Verification items for the finished model (mm, model axes). Give positions to 0.01 mm unless a question says otherwise; leave off trailing zeros. Write each loop counter-clockwise with the first axis right and the second up, starting at its lowest first coordinate (ties: lowest second). Pieces come first, ordered by that corner, then holes. Notation, with made-up numbers: (84.25, 58) -> (108.25, 58) arc R21 ccw to (108.25, 89) -> close; hole circle Ø7 at (-24.5, 41). An arc over 180 degrees is marked (long way). Write item = value, one per line.
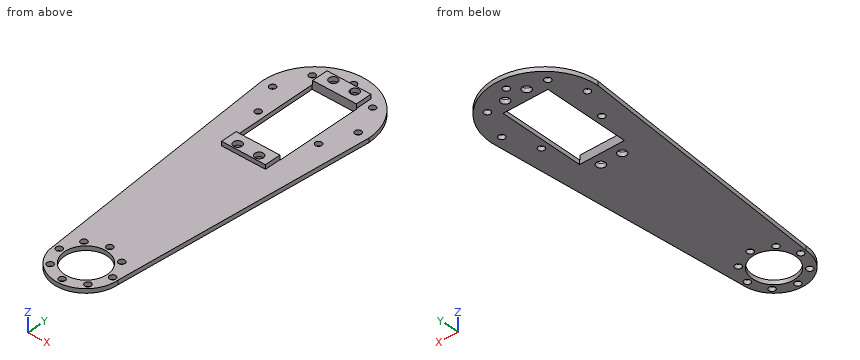
from build123d import *

# Parameters (mm, degrees)
SKETCH_1_W          = 20.5
SKETCH_1_H          = 15.141704846
SKETCH_1_R          = 2
EXTRUDE_1_DEPTH     = 29
SKETCH_2_W          = 20.5
SKETCH_2_H          = 70.283409692
EXTRUDE_2_DEPTH     = 3
SKETCH_3_W          = 20.5
SKETCH_3_H          = 7.570852423
CUT_EXTRUDE_1_DEPTH = 49.621002864
SKETCH_5_R          = 2.5
EXTRUDE_3_DEPTH     = 10
CUT_EXTRUDE_2_REACH = 75.297
SKETCH_8_R          = 1.6
SKETCH_9_W          = 20.5
SKETCH_9_H          = 55.141704846
CUT_EXTRUDE_3_DEPTH = 30
SKETCH_11_R         = 2.5
CUT_EXTRUDE_4_DEPTH = 10
SKETCH_12_W         = 21
SKETCH_12_H         = 40
SKETCH_12_R         = 2
EXTRUDE_5_DEPTH     = 2
SKETCH_13_R         = 10
CUT_EXTRUDE_5_DEPTH = 2
SKETCH_14_R         = 1.5
CUT_EXTRUDE_6_DEPTH = 128.538229563


with BuildPart() as part:
    # Sketch 1 → Extrude 1 (new body)
    # profile 1 of 3: a face of its own
    with BuildSketch(Plane.XY):
        with BuildLine():
            Line((-10.25, 35.141704846), (-10.25, 20))
            Line((-10.25, 20), (-5, 20))
            Line((-5, 20), (-5, 23))
            ThreePointArc((-5, 23), (-6.414213562, 26.414213562), (-3, 25))
            Line((-3, 25), (3, 25))
            ThreePointArc((3, 25), (5, 27), (7, 25))
            ThreePointArc((7, 25), (6.414213562, 23.585786438), (5, 23))
            Line((5, 23), (5, 20))
            Line((5, 20), (10.25, 20))
            Line((10.25, 20), (10.25, 35.141704846))
            Line((10.25, 35.141704846), (-10.25, 35.141704846))
        make_face()
    # profile 2 of 3: a face of its own
    with BuildSketch(Plane.XY):
        with Locations((0, -27.570852423)):
            Rectangle(SKETCH_1_W, SKETCH_1_H)
        with Locations(Location((-5, -25, 0), (0, 0, 180))):
            Circle(SKETCH_1_R, mode=Mode.SUBTRACT)
        with Locations(Location((5, -25, 0), (0, 0, 180))):
            Circle(SKETCH_1_R, mode=Mode.SUBTRACT)
    # profile 3 of 3: a face of its own
    with BuildSketch(Plane.XY):
        with BuildLine():
            Line((-5, 23), (-5, 20))
            Line((-5, 20), (5, 20))
            Line((5, 20), (5, 23))
            ThreePointArc((5, 23), (3.585786438, 23.585786438), (3, 25))
            Line((3, 25), (-3, 25))
            ThreePointArc((-3, 25), (-3.585786438, 23.585786438), (-5, 23))
        make_face()
    extrude(amount=EXTRUDE_1_DEPTH)

    # Sketch 2 → Extrude 2 (add)
    with BuildSketch(Plane.XY.offset(29)):
        Rectangle(SKETCH_2_W, SKETCH_2_H)
    extrude(amount=EXTRUDE_2_DEPTH)

    # Sketch 3 → Cut-Extrude 1 (cut, through all)
    with BuildSketch(Plane(origin=(0, 0, 0), x_dir=(-1, 0, 0), z_dir=(0, 0, -1))):
        with Locations((0, -31.356278635)):
            Rectangle(SKETCH_3_W, SKETCH_3_H)
        with Locations((0, 31.356278635)):
            Rectangle(SKETCH_3_W, SKETCH_3_H)
    extrude(amount=-CUT_EXTRUDE_1_DEPTH, mode=Mode.SUBTRACT)

    # Sketch 5 → Extrude 3 (add)
    with BuildSketch(Plane.XZ.offset(27.570852423)):
        with Locations(Location((0, 2.5, 0), (0, 0, 270))):
            Circle(SKETCH_5_R)
    extrude(amount=EXTRUDE_3_DEPTH)

    # Sketch 8 → Cut-Extrude 2 (cut, up to next)
    with BuildSketch(Plane(origin=(0, 27.570852423, 0), x_dir=(1, 0, 0), z_dir=(0, 1, 0)), mode=Mode.PRIVATE) as cut_extrude_2_sk1:
        with Locations(Location((0, -16.5, 0), (0, 0, 270))):
            Circle(SKETCH_8_R)
    cut_extrude_2_tool1 = extrude(cut_extrude_2_sk1.sketch, amount=-CUT_EXTRUDE_2_REACH, mode=Mode.PRIVATE) & part.part
    # Sketch 8 → Cut-Extrude 2 (cut, up to next)
    with BuildSketch(Plane(origin=(0, 27.570852423, 0), x_dir=(1, 0, 0), z_dir=(0, 1, 0)), mode=Mode.PRIVATE) as cut_extrude_2_sk2:
        with Locations(Location((0, -26.5, 0), (0, 0, 270))):
            Circle(SKETCH_8_R)
    cut_extrude_2_tool2 = extrude(cut_extrude_2_sk2.sketch, amount=-CUT_EXTRUDE_2_REACH, mode=Mode.PRIVATE) & part.part
    add(cut_extrude_2_tool1.solids().sort_by_distance((0, 27.570852, 16.5))[0], mode=Mode.SUBTRACT)
    add(cut_extrude_2_tool2.solids().sort_by_distance((0, 27.570852, 26.5))[0], mode=Mode.SUBTRACT)

    # Sketch 9 → Cut-Extrude 3 (cut)
    with BuildSketch(Plane.XY.offset(32)):
        Rectangle(SKETCH_9_W, SKETCH_9_H)
    extrude(amount=-CUT_EXTRUDE_3_DEPTH, mode=Mode.SUBTRACT)


with BuildPart() as cut_extrude_3_piece_1:
    # of the separate pieces the step leaves, piece 1, a body of its own (cut_extrude_3_pieces)
    add(part.part.solids().sort_by_distance((10.25, -20, 2))[0])

    # Sketch 11 → Cut-Extrude 4 (cut)
    with BuildSketch(Plane.XZ.offset(37.570852423)):
        with Locations((0, 2.5)):
            Circle(SKETCH_11_R)
    extrude(amount=-CUT_EXTRUDE_4_DEPTH, mode=Mode.SUBTRACT)



with BuildPart() as cut_extrude_3_piece_2:
    # of the separate pieces the step leaves, piece 2, a body of its own (cut_extrude_3_pieces)
    add(part.part.solids().sort_by_distance((10.25, 20, 0))[0])


with BuildPart() as cut_extrude_3_piece_1_1:
    add(cut_extrude_3_piece_1.part)

    add(cut_extrude_3_piece_2.part)  # Extrude 5 merges Cut-Extrude 3 piece 2
    # Sketch 12 → Extrude 5 (add)
    with BuildSketch(Plane(origin=(0, 0, 0), x_dir=(-1, 0, 0), z_dir=(0, 0, -1))):
        with BuildLine():
            Line((15, -110), (25, 10))
            ThreePointArc((25, 10), (0, 35), (-25, 10))
            Line((-25, 10), (-15, -110))
            ThreePointArc((-15, -110), (0, -125), (15, -110))
        make_face()
        Rectangle(SKETCH_12_W, SKETCH_12_H, mode=Mode.SUBTRACT)
        with Locations((-5, 25)):
            Circle(SKETCH_12_R, mode=Mode.SUBTRACT)
        with Locations((5, 25)):
            Circle(SKETCH_12_R, mode=Mode.SUBTRACT)
        with Locations(Location((5, -25, 0), (0, 0, 180))):
            Circle(SKETCH_12_R, mode=Mode.SUBTRACT)
        with Locations(Location((-5, -25, 0), (0, 0, 180))):
            Circle(SKETCH_12_R, mode=Mode.SUBTRACT)
    extrude(amount=EXTRUDE_5_DEPTH)

    # Sketch 13 → Cut-Extrude 5 (cut)
    with BuildSketch(Plane(origin=(0, 0, -2), x_dir=(-1, 0, 0), z_dir=(0, 0, -1))):
        with Locations((0, -110)):
            Circle(SKETCH_13_R)
    extrude(amount=-CUT_EXTRUDE_5_DEPTH, mode=Mode.SUBTRACT)

    # Sketch 14 → Cut-Extrude 6 (cut, through all)
    with BuildSketch(Plane(origin=(0, 0, -2), x_dir=(-1, 0, 0), z_dir=(0, 0, -1))):
        with Locations((-20, 10)):
            Circle(SKETCH_14_R)
        with Locations((-14.142135624, 24.142135624)):
            Circle(SKETCH_14_R)
        with Locations((0, 30)):
            Circle(SKETCH_14_R)
        with Locations((14.142135624, 24.142135624)):
            Circle(SKETCH_14_R)
        with Locations((20, 10)):
            Circle(SKETCH_14_R)
        with Locations((14.142135624, -4.142135624)):
            Circle(SKETCH_14_R)
        with Locations((-14.142135624, -4.142135624)):
            Circle(SKETCH_14_R)
        with Locations((0, -97.5)):
            Circle(SKETCH_14_R)
        with Locations((8.838834765, -101.161165235)):
            Circle(SKETCH_14_R)
        with Locations((12.5, -110)):
            Circle(SKETCH_14_R)
        with Locations((8.838834765, -118.838834765)):
            Circle(SKETCH_14_R)
        with Locations((0, -122.5)):
            Circle(SKETCH_14_R)
        with Locations((-8.838834765, -118.838834765)):
            Circle(SKETCH_14_R)
        with Locations((-12.5, -110)):
            Circle(SKETCH_14_R)
        with Locations((-8.838834765, -101.161165235)):
            Circle(SKETCH_14_R)
    extrude(amount=-CUT_EXTRUDE_6_DEPTH, mode=Mode.SUBTRACT)


solid = cut_extrude_3_piece_1_1.part
Item 1: Material ranges on line 1 (Y direction, x = 5, z = 0.8); line 2 (Y direction, x = 0, z = -1.2); line 3 (X direction, y = -24, z = -1.75), recorded low to high.
Response values:
line_1 = -27.57 to -27, -23 to -20, 20 to 23, 27 to 27.57
line_2 = -125 to -124, -121 to -120, -100 to -99, -96 to -20, 20 to 28.5, 31.5 to 35
line_3 = -22.17 to -6.73, -3.27 to 3.27, 6.73 to 22.17
Item 2: Sectioned sample at D-D on z = -0.75. Give the number of separate pieces and of enclosed holes in the cut face, then the cut area to 3 significant figures.
Response values:
separate_pieces = 1
enclosed_holes = 21
area = 4,820 mm^2
Item 3: Sectioned sample at A-A on x = 0. Record the cut outline in (y, z), then the cut area to 3 significant figures.
Response values:
outline = (-125, -2) -> (-124, -2) -> (-124, 0) -> (-125, 0) -> close; (-121, -2) -> (-120, -2) -> (-120, 0) -> (-121, 0) -> close; (-100, -2) -> (-99, -2) -> (-99, 0) -> (-100, 0) -> close; (-96, -2) -> (-20, -2) -> (-20, 2) -> (-27.57, 2) -> (-27.57, 0) -> (-96, 0) -> close; (20, -2) -> (28.5, -2) -> (28.5, 0) -> (27.57, 0) -> (27.57, 2) -> (20, 2) -> close; (31.5, -2) -> (35, -2) -> (35, 0) -> (31.5, 0) -> close
area = 212 mm^2
Item 4: Go/stop test with flat-tipped pins: P1, Ø5, axis at x = 5, y = -25, coming from the -Z side; P2, Ø1.2, axis at x = 2.5, z = 0, coming from the +Y side; P3, Ø1, axis at x = -2.5, z = 1, coming from the -Y side; P4, Ø1.6, axis at y = -23, z = 1, coming from the +X side. Record where each tip stops, or that it passes through.
Response values:
P1 = -2
P2 = 34.93
P3 = -27.57
P4 = 10.25
Item 5: Sectioned sample at C-C on x = -20. Record the cut outline in (y, z).
Response values:
outline = (-50, -2) -> (8.5, -2) -> (8.5, 0) -> (-50, 0) -> close; (11.5, -2) -> (25, -2) -> (25, 0) -> (11.5, 0) -> close
Item 6: Sectioned sample at B-B on y = -122.5. Record the cut outline in (x, z).
Response values:
outline = (-8.29, -2) -> (-1.5, -2) -> (-1.5, 0) -> (-8.29, 0) -> close; (1.5, -2) -> (8.29, -2) -> (8.29, 0) -> (1.5, 0) -> close
